Here's how the part is built. I have some questions about the finished solid (model axes, mm). Face numbers are marked on the shaded views. A direction names the side the tool comes from. Round coordinates to 2 decimals unless told otherwise and drop trailing zeros. Order: outer loops, then holes, each group sorted by start corner. A loop starts at its lowest first (then second) coordinate and runs counter-clockwise, first axis right, second up. Notation, with made-up numbers: (47.25, 11.25) -> (55.25, 11.25) arc R19 cw to (55.25, 26.25) -> close; hole circle Ø9 at (41, 28). An arc over 180 degrees is marked (long way). Answer in a Markdown table with one row per item.
```python
from build123d import *

# Parameters (mm, degrees)
BOX017_W        = 10
BOX017_H        = 5
BOX017_DEPTH    = 10
CHAMFER006_SIZE = 2
BOX016_W        = 10
BOX016_H        = 5
BOX016_DEPTH    = 10
CHAMFER007_SIZE = 1


with BuildPart() as chamfer014:
    # Box017 → Box017 (new body)
    with BuildSketch(Plane(origin=(-2, 0, 2), x_dir=(1, 0, 0), z_dir=(0, 0, 1))):
        with Locations((5, 2.5)):
            Rectangle(BOX017_W, BOX017_H)
    extrude(amount=BOX017_DEPTH)

    # Chamfer006
    chamfer006_edges = [chamfer014.edges().sort_by_distance(p)[0] for p in [
        (8, 2.5, 2),
    ]]
    chamfer(chamfer006_edges, length=CHAMFER006_SIZE)


with BuildPart() as obj1:
    # Box016 → Box016 (new body)
    with BuildSketch(Plane.XY):
        with Locations((5, 2.5)):
            Rectangle(BOX016_W, BOX016_H)
    extrude(amount=BOX016_DEPTH)

    # Cut001017: cut Chamfer014
    add(chamfer014.part, mode=Mode.SUBTRACT)

    # Chamfer007
    chamfer007_edges = [obj1.edges().sort_by_distance(p)[0] for p in [
        (10, 2.5, 0),
    ]]
    chamfer(chamfer007_edges, length=CHAMFER007_SIZE)


with BuildPart() as obj1_1:
    # Chamfer007 placement: moved
    add(obj1.part.moved(Location((-23, 0, 0))))


solid = obj1_1.part
```
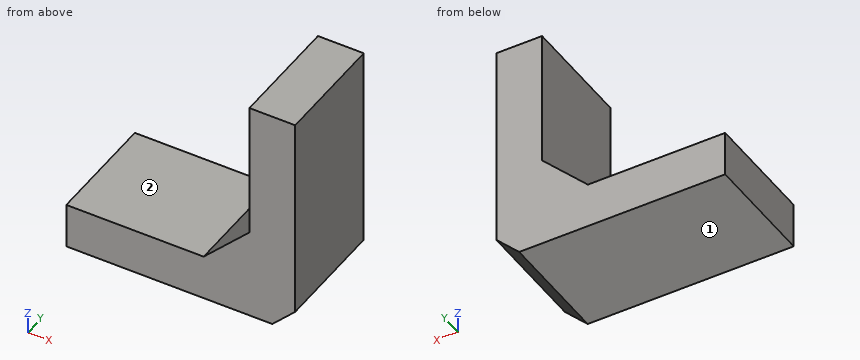
1. For pin 1 Ø2 at (x, y) = (-19, 3.5) entering from +Z, with a flat end and sliding along its axis, tell me the tip position at first contact or that it passes through.
Numbers:
| item | result |
|---|---|
| pin 1 | stops at z = 2 |
2. Suppose I cut it at C-C on x = -15.75. Write out the boundary of the cut face in (y, z).
Numbers:
| item | result |
|---|---|
| outline | (0, 0) -> (5, 0) -> (5, 3.25) -> (0, 3.25) -> close |
3. Please list where these lines run through material, in increasing order: line 1 along Z through (x, y) = (-21.75, 3.3); line 2 along X through (y, z) = (3.75, 5.5); line 3 along Z through (x, y) = (-16, 3.15).
Numbers:
| item | result |
|---|---|
| line 1 | z = 0 to 2 |
| line 2 | x = -15 to -13 |
| line 3 | z = 0 to 3 |
4. Suppose I cut it at A-A on y = 3.9. Write out the boundary of the cut face in (x, z), then the cut area to 3 significant figures.
Numbers:
| item | result |
|---|---|
| outline | (-23, 0) -> (-14, 0) -> (-13, 1) -> (-13, 10) -> (-15, 10) -> (-15, 4) -> (-17, 2) -> (-23, 2) -> close |
| area | 37.5 mm2 |
5. For the marked faces 1 and 2, which set-ups out of +Z, -Z, +X, -X, +Y, -Y let a thin tool reach every point of the face, with its end or its side?
Numbers:
| item | result |
|---|---|
| face 1 | -Z, +X, -X, +Y, -Y |
| face 2 | +Z, -X, +Y, -Y |
6. Suppose I cut it at B-B on z = 7.25. Write out the boundary of the cut face in (x, y).
Numbers:
| item | result |
|---|---|
| outline | (-15, 0) -> (-13, 0) -> (-13, 5) -> (-15, 5) -> close |
